Geometry check sheet. Reference: the model listing, model coordinates, mm. Face numbers are marked on the shaded views. A direction names the side the tool comes from. Round coordinates to 2 decimals unless told otherwise and drop trailing zeros. Order: outer loops, then holes, each group sorted by start corner. A loop starts at its lowest first (then second) coordinate and runs counter-clockwise, first axis right, second up. Notation, with made-up numbers: (-8, 73) - (16, 73) arc R15 ccw to (16, 91) - close; hole circle Ø8 at (-9, -22.5). An arc over 180 degrees is marked (long way). Use a Markdown table: item, result. Add a question column.
(1) Section check B-B on z = -1.75. Record the boundary of the cut face in (x, y), then the cut area to 3 significant figures.
(2) Section check D-D on y = 7.5. Record the boundary of the cut face in (x, z), then the cut area to 3 significant figures.
(3) Gauge pin test, flat ends, axial feed: P1, Ø1.5, axis at y = 4, z = -1, coming from the -X side; P2, Ø2, axis at x = -2.5, y = 10.5, coming from the +Z side; P3, Ø5, axis at x = -5, y = 6, coming from the +Z side. Record the tip position at first contact, or that the pin passes through.
(4) Access from +Z, -Z, +X, -X, +Y, -Y to the whole of each face (thin tool, end or side, straight path). Record for the marked faces 4, 5 and 6.
(5) Thickness scan on line 1 along Y through (x, z) = (-4.5, 8.75); line 2 along X through (y, z) = (1.75, 5.75); line 3 along X through (y, z) = (8.5, 2.5). Record the ranges inside material, lowest first. Write a range as [from, to].
(6) Mould release check, pull along X, two halves, no side actions. Record for the marked faces 1, 2 and 3: released by +X, released by -X, zero draft, split by the parting line, or undercut.
(7) Section check A-A on x = -6. Record the boundary of the cut face in (y, z).
(8) Section check C-C on y = 3. Record the boundary of the cut face in (x, z), then the cut area to 3 significant figures.
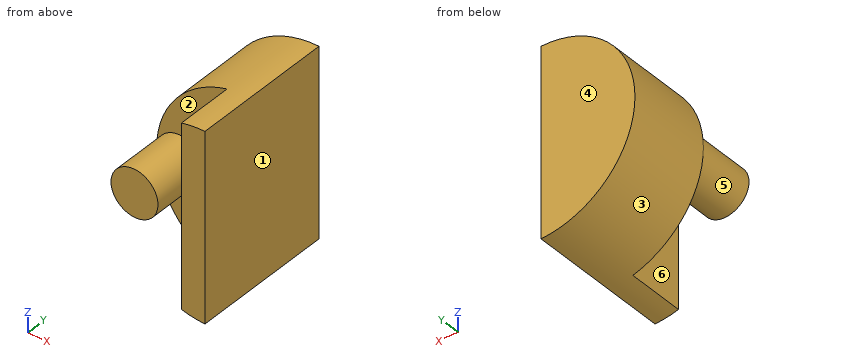
```python
from build123d import *

# Parameters (mm, degrees)
SALIENTE_EXTRUIR1_DEPTH = 15
CROQUIS2_W              = 7.5
CROQUIS2_H              = 6
CORTAR_EXTRUIR2_DEPTH   = 27.925824036
CROQUIS4_R              = 2.5
SALIENTE_EXTRUIR2_DEPTH = 6


with BuildPart() as part:
    # Croquis1 → Saliente-Extruir1 (new body)
    with BuildSketch(Plane(origin=(0, 0, 0), x_dir=(1, 0, 0), z_dir=(0, 1, 0))):
        with BuildLine():
            Line((0, 10), (0, -10))
            ThreePointArc((0, -10), (-10, 0), (0, 10))
        make_face()
    extrude(amount=SALIENTE_EXTRUIR1_DEPTH)

    # Croquis2 → Cortar-Extruir2 (cut, through all)
    with BuildSketch(Plane.XY.offset(10)):
        with Locations((-6.25, 3)):
            Rectangle(CROQUIS2_W, CROQUIS2_H)
    extrude(amount=-CORTAR_EXTRUIR2_DEPTH, mode=Mode.SUBTRACT)

    # Croquis4 → Saliente-Extruir2 (add)
    with BuildSketch(Plane.XZ.offset(-6)):
        with Locations(Location((-7.5, 0, 0), (0, 0, 179.999408267))):
            Circle(CROQUIS4_R)
    extrude(amount=SALIENTE_EXTRUIR2_DEPTH)


solid = part.part
```
Check sheet entries:
| question | item | result |
|---|---|---|
| 1 | outline | (-9.85, 6) - (-9.29, 6) - (-9.29, 0) - (-5.71, 0) - (-5.71, 6) - (-2.5, 6) - (-2.5, 0) - (0, 0) - (0, 15) - (-9.85, 15) - close |
| 1 | area | 125 mm2 |
| 2 | outline | (0, -10) - (0, 10) arc R10 ccw to start |
| 2 | area | 157 mm2 |
| 3 | P1 | stops at x = -9.99 |
| 3 | P2 | stops at z = 9.89 |
| 3 | P3 | stops at z = 9.68 |
| 4 | face 4 | +Z, -Z, +X, -X, +Y |
| 4 | face 5 | -Y |
| 4 | face 6 | +Z, -Z, -Y |
| 5 | line 1 | y = [6, 15] |
| 5 | line 2 | x = [-2.5, 0] |
| 5 | line 3 | x = [-9.68, 0] |
| 6 | face 1 | released by +X |
| 6 | face 2 | undercut |
| 6 | face 3 | released by -X |
| 7 | outline | (0, -2) - (6, -2) - (6, -8) - (15, -8) - (15, 8) - (6, 8) - (6, 2) - (0, 2) - close |
| 8 | outline | circle Ø5 at (-7.5, 0); (-2.5, -9.68) arc R10 ccw to (0, -10) - (0, 10) arc R10 ccw to (-2.5, 9.68) - close |
| 8 | area | 69.1 mm2 |
